```python
from build123d import *

# Parameters (mm, degrees)
F0_R     = 1.5875
F1_DEPTH = 3.175
F3_DEPTH = 1.5875
F4_SIZE  = 2.54


with BuildPart() as f1:
    # F0 (on Top) → F1 (new body)
    with BuildSketch(Plane.XY):
        with BuildLine():
            ThreePointArc((-38.094764, -12.153731), (-36.234892, -16.643859), (-31.744764, -18.503731))
            Line((-31.744764, -18.503731), (-19.044764, -18.503731))
            ThreePointArc((-19.044764, -18.503731), (-14.554635, -16.643859), (-12.694764, -12.153731))
            Line((-12.694764, -12.153731), (-12.694764, 51.346269))
            ThreePointArc((-12.694764, 51.346269), (-14.554635, 55.836397), (-19.044764, 57.696269))
            Line((-19.044764, 57.696269), (-31.744764, 57.696269))
            ThreePointArc((-31.744764, 57.696269), (-36.234892, 55.836397), (-38.094764, 51.346269))
            Line((-38.094764, 51.346269), (-38.094764, -12.153731))
        make_face()
        with BuildLine():
            Line((-29.952724, 13.335001), (-30.358404, 13.335001))
            Line((-30.358404, 13.335001), (-30.358404, -7.376809))
            Line((-30.358404, -7.376809), (-34.330532, -7.376809))
            Line((-34.330532, -7.376809), (-34.330532, 13.335001))
            ThreePointArc((-34.330532, 13.335001), (-25.393245, 22.272288), (-16.455958, 13.335001))
            Line((-16.455958, 13.335001), (-16.455958, -7.376809))
            Line((-16.455958, -7.376809), (-20.711809, -7.376809))
            Line((-20.711809, -7.376809), (-20.711809, 13.335001))
            Line((-20.711809, 13.335001), (-20.833766, 13.335001))
            ThreePointArc((-20.833766, 13.335001), (-25.393245, 17.89448), (-29.952724, 13.335001))
        make_face(mode=Mode.SUBTRACT)
        with Locations((-25.394764, 44.940945)):
            Circle(F0_R, mode=Mode.SUBTRACT)
    extrude(amount=F1_DEPTH)

    # F2 (on face) → F3 (join)
    with BuildSketch(Plane.XY.offset(3.175)):
        with BuildLine():
            ThreePointArc((-29.987899, 13.335001), (-25.393245, 8.740347), (-20.798591, 13.335001))
            Line((-20.798591, 13.335001), (-20.833766, 13.335001))
            ThreePointArc((-20.833766, 13.335001), (-25.393245, 17.89448), (-29.952724, 13.335001))
            Line((-29.952724, 13.335001), (-29.987899, 13.335001))
        make_face()
    extrude(amount=F3_DEPTH)

    # F4
    f4_edges = [f1.edges().sort_by_distance(p)[0] for p in [
        (-26.982264, 44.940945, 3.175),
    ]]
    chamfer(f4_edges, length=F4_SIZE)


solid = f1.part
```
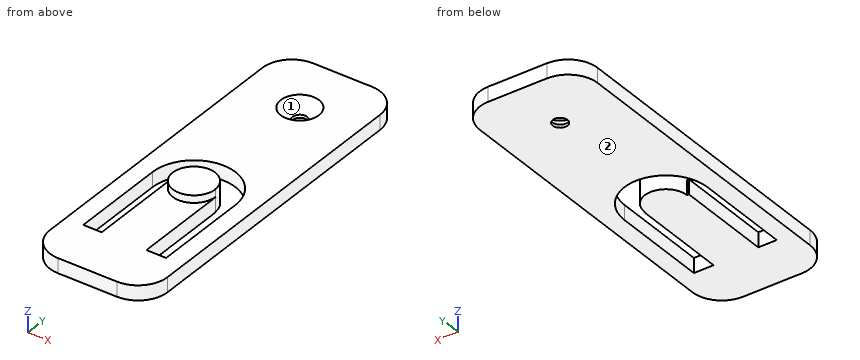
Geometry check sheet. Reference: the model listing, model coordinates, mm. Face numbers are marked on the shaded views. Round coordinates to 2 decimals unless told otherwise and drop trailing zeros. Order: outer loops, then holes, each group sorted by start corner. A loop starts at its lowest first (then second) coordinate and runs counter-clockwise, first axis right, second up. Notation, with made-up numbers: (28, -10) - (60, -10) arc R10 ccw to (60, -2) - close; hole circle Ø4 at (7, 88). An arc over 180 degrees is marked (long way). Use a Markdown table: item, result. Add a question column.
(1) Sectioned sample at B-B, the plane x = -17.5. Enter the section's corners in (y, z) (1 decimal), and give its area (3 significant figures).
(2) Sectioned sample at A-A, the plane y = 7. Enter the section's corners in (x, z) (3 decimals).
(3) Material ranges on line 1 along X through (y, z) = (7, 3); line 2 along X through (y, z) = (16, 1.1); line 3 along Y through (x, z) = (-26.75, 0.5), recorded low to high. Write a range as [from, to].
(4) Sectioned sample at D-D, the plane y = 15. Enter the section's corners in (x, z) (1 decimal), and give its area (3 significant figures).
(5) Sectioned sample at C-C, the plane z = 1.5. Count the separate pieces of the cut face and the enclosed holes in it, and give its area (3 significant figures).
(6) Depth check by flat-ended pin: pin 1 (2.5 mm diameter, centred on x = -17.5, z = 1.5, fed in from +Y); pin 2 (1.5 mm diameter, centred on x = -15.5, z = 4, fed in from -Y); pin 3 (4 mm diameter, centred on x = -25.39, y = 44.94, fed in from +Z). Enter the tip coordinate at first touch or a pass-through.
(7) Release check for a two-part mould opening along Y. For the marked faces 1 and 2 record: pulls with the +Y half, pulls with the -Y half, needs draft (parallel to the pull), parting line crosses it, or undercut.
Answers below:
| question | item | result |
|---|---|---|
| 1 | outline | (-18.3, 0) - (-7.4, 0) - (-7.4, 3.2) - (-18.3, 3.2) - close; (17.5, 0) - (57.5, 0) - (57.5, 3.2) - (17.5, 3.2) - close |
| 1 | area | 162 mm² |
| 2 | outline | (-38.095, 0) - (-34.331, 0) - (-34.331, 3.175) - (-38.095, 3.175) - close; (-30.358, 0) - (-20.712, 0) - (-20.712, 3.175) - (-30.358, 3.175) - close; (-16.456, 0) - (-12.695, 0) - (-12.695, 3.175) - (-16.456, 3.175) - close |
| 3 | line 1 | [-38.09, -34.33], [-30.36, -20.71], [-16.46, -12.69] |
| 3 | line 2 | [-38.09, -33.92], [-29.09, -21.69], [-16.86, -12.69] |
| 3 | line 3 | [-18.5, 17.69], [22.17, 44.11], [45.77, 57.7] |
| 4 | outline | (-38.1, 0) - (-34.2, 0) - (-34.2, 3.2) - (-38.1, 3.2) - close; (-29.6, 0) - (-21.1, 0) - (-21.1, 4.8) - (-29.6, 4.8) - close; (-16.6, 0) - (-12.7, 0) - (-12.7, 3.2) - (-16.6, 3.2) - close |
| 4 | area | 65.3 mm² |
| 5 | separate pieces | 1 |
| 5 | enclosed holes | 2 |
| 5 | area | 1,620 mm² |
| 6 | pin 1 | y = 57.69 |
| 6 | pin 2 | through |
| 6 | pin 3 | z = 1.05 |
| 7 | face 1 | undercut |
| 7 | face 2 | needs draft |
